from build123d import *

# Parameters (mm, degrees)
SKETCH_1_W          = 65
SKETCH_1_H          = 15
EXTRUDE_1_DEPTH     = 2
FILLET_1_R          = 7.5
SKETCH_2_R          = 2
SKETCH_2_R_2        = 1
CUT_EXTRUDE_1_DEPTH = 10
SKETCH_4_R          = 1.25
CUT_EXTRUDE_3_DEPTH = 10
SKETCH_8_R          = 1.25
CUT_EXTRUDE_6_DEPTH = 10
SKETCH_9_W          = 8
SKETCH_9_H          = 4.970258762
CUT_EXTRUDE_7_DEPTH = 10
SKETCH_10_W         = 8.5
SKETCH_10_H         = 5
CUT_EXTRUDE_8_DEPTH = 2
FILLET_3_R          = 2


with BuildPart() as part:
    # 草图1 → 凸台-拉伸1 (new body)
    with BuildSketch(Plane.XY):
        Rectangle(SKETCH_1_W, SKETCH_1_H)
    extrude(amount=EXTRUDE_1_DEPTH)

    # 圆角1
    fillet_1_edges = [part.edges().sort_by_distance(p)[0] for p in [
        (32.5, 7.5, 1),
        (32.5, -7.5, 1),
    ]]
    fillet(fillet_1_edges, radius=FILLET_1_R - 0.0001)  # a hair under: the kernel refuses the full size

    # 草图2 → 切除-拉伸1 (cut)
    with BuildSketch(Plane.XY.offset(2)):
        with Locations((25, 0)):
            Circle(SKETCH_2_R)
        with Locations((-25, 5)):
            Circle(SKETCH_2_R_2)
        with Locations((-10, 5)):
            Circle(SKETCH_2_R_2)
    extrude(amount=-CUT_EXTRUDE_1_DEPTH, mode=Mode.SUBTRACT)

    # 草图4 → 切除-拉伸3 (cut)
    with BuildSketch(Plane(origin=(0, 0, 0), x_dir=(-1, 0, 0), z_dir=(0, 0, -1))):
        with Locations((21.5, -3.5)):
            Circle(SKETCH_4_R)
        with Locations((13.5, -3.5)):
            Circle(SKETCH_4_R)
    extrude(amount=-CUT_EXTRUDE_3_DEPTH, mode=Mode.SUBTRACT)

    # 草图8 → 切除-拉伸6 (cut)
    with BuildSketch(Plane.XY.offset(2)):
        with Locations((7.5, 0.5)):
            Circle(SKETCH_8_R)
        with Locations((1.5, 0.5)):
            Circle(SKETCH_8_R)
    extrude(amount=-CUT_EXTRUDE_6_DEPTH, mode=Mode.SUBTRACT)

    # 草图9 → 切除-拉伸7 (cut)
    with BuildSketch(Plane.XY.offset(2)):
        with Locations((-17.5, 5.014870619)):
            Rectangle(SKETCH_9_W, SKETCH_9_H)
    extrude(amount=-CUT_EXTRUDE_7_DEPTH, mode=Mode.SUBTRACT)

    # 草图10 → 切除-拉伸8 (cut)
    with BuildSketch(Plane.XY.offset(2)):
        with Locations((-28.25, -5)):
            Rectangle(SKETCH_10_W, SKETCH_10_H)
    extrude(amount=-CUT_EXTRUDE_8_DEPTH, mode=Mode.SUBTRACT)

    # 圆角3
    fillet_3_edges = [part.edges().sort_by_distance(p)[0] for p in [
        (-21.5, 2.529741238, 1),
        (-21.5, 7.5, 1),
        (-13.5, 7.5, 1),
        (-13.5, 2.529741238, 1),
        (-32.5, 7.5, 1),
        (-32.5, -2.5, 1),
        (-24, -2.5, 1),
        (-24, -7.5, 1),
    ]]
    fillet(fillet_3_edges, radius=FILLET_3_R)


solid = part.part
Model file for the job. Use its own axes, mm. A direction names the side the tool comes from. Round coordinates to 2 decimals unless told otherwise and drop trailing zeros. Loops run counter-clockwise (first coordinate to the right, second up) from the corner with the lowest first, then second, coordinate; pieces in that order, holes last. Notation, with made-up numbers: (58, 75.25) -> (81, 75.25) arc R9 ccw to (81, 80.25) -> close; hole circle Ø4 at (55.5, 34). An arc over 180 degrees is marked (long way). Answer as CSV lines item,"result". Start each with the question number.
1) Slice it at D-D (x = -10). List the corners of the cut face in (y, z).
2) Slice it at B-B (z = 0.45). State how many separate pieces and enclosed holes the cut face has, plus the area to 3 significant figures.
3) Slice it at C-C (y = -3.5). List the corners of the cut face in (x, z).
4) Probe line 1 along Y through (x, z) = (-10, 0.4); line 2 along X through (y, z) = (1, 0.45); line 3 along X through (y, z) = (4.25, 0.45). List the from-to ranges inside material, lowest first.
5) Tool access for faces 1 (the face through (-28, -2.5, 1)), 2 (the face through (-27, 7.5, 1)), 3 (the face through (-18, 2.53, 1)): list every direction of +Z, -Z, +X, -X, +Y, -Y with a clear straight run to the whole face (end or side of a thin tool).
6) Mould opens along X. For faces 4 (the face through (0, 0, 2)), 5 (the face through (30.361, 5.245, 1.014)), 6 (the face through (1.34, 1.74, 1.01)) say: +X half, -X half, draft (parallel to the pull), parting line (faces both ways), or undercut.
7) Slice it at A-A (x = 7.5). List the corners of the cut face in (y, z), plus the area to 3 significant figures.
8) Pin check, flat tips, straight feed: P1, Ø1.1, axis at y = -5, z = 0.5, coming from the -X side; P2, Ø1.5, axis at x = -21.5, y = -3.5, coming from the -Z side. Stop position of each tip, or through.
Filled in:
1,outline,"(-7.5, 0) -> (4, 0) -> (4, 2) -> (-7.5, 2) -> close; (6, 0) -> (7.5, 0) -> (7.5, 2) -> (6, 2) -> close"
2,separate pieces,"1"
2,enclosed holes,"7"
2,area,"828 mm2"
3,outline,"(-24.27, 0) -> (-22.75, 0) -> (-22.75, 2) -> (-24.27, 2) -> close; (-20.25, 0) -> (-14.75, 0) -> (-14.75, 2) -> (-20.25, 2) -> close; (-12.25, 0) -> (31.63, 0) -> (31.63, 2) -> (-12.25, 2) -> close"
4,line 1,"y = -7.5 to 4, 6 to 7.5"
4,line 2,"x = -32.5 to 0.35, 2.65 to 6.35, 8.65 to 23.27, 26.73 to 32.43"
4,line 3,"x = -32.5 to -25.66, -24.34 to -21.48, -13.52 to -10.66, -9.34 to 31.18"
5,face 1,"+Z, -Z, -X, -Y"
5,face 2,"+Z, -Z, +X, -X, +Y"
5,face 3,"+Z, -Z, +Y"
6,face 4,"draft"
6,face 5,"+X half"
6,face 6,"undercut"
7,outline,"(-7.5, 0) -> (-0.75, 0) -> (-0.75, 2) -> (-7.5, 2) -> close; (1.75, 0) -> (7.5, 0) -> (7.5, 2) -> (1.75, 2) -> close"
7,area,"25.0 mm2"
8,P1,"stops at x = -24"
8,P2,"passes through"
